Check sheet for the drawn part. Datum: minimum x, y, z corner. Units: mm. A direction names the side the tool comes from. Round coordinates to 2 decimals unless told otherwise and drop trailing zeros. Loops run counter-clockwise (first coordinate to the right, second up) from the corner with the lowest first, then second, coordinate; pieces in that order, holes last. Notation, with made-up numbers: (84.25, 70) - (90.25, 70) arc R27 cw to (90.25, 99) - close; hole circle Ø2 at (86, -19.75). An arc over 180 degrees is marked (long way). Use CSV: the item, a comma, the result in double quotes.
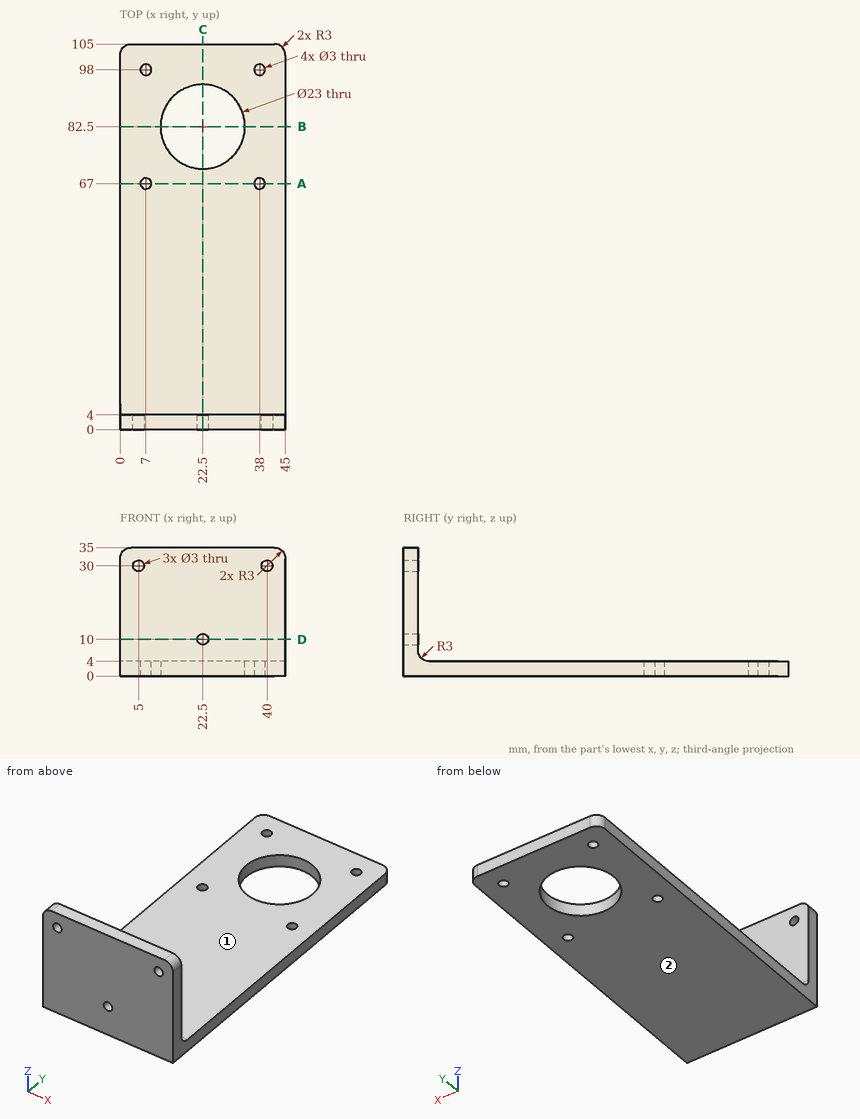
1) Cross-section at D-D, the plane z = 10. Record the cut outline in (x, y), then the cut area to 3 significant figures.
Returned:
outline,"(0, 0) - (21, 0) - (21, 4) - (0, 4) - close; (24, 0) - (45, 0) - (45, 4) - (24, 4) - close"
area,"168 mm²"
2) Access from +Z, -Z, +X, -X, +Y, -Y to the whole of each face (thin tool, end or side, straight path). Record for the marked faces 1 and 2.
Returned:
face 1,"+Z, +X, -X, +Y"
face 2,"-Z, +X, -X, +Y, -Y"
3) Cross-section at C-C, the plane x = 22.5. Record the cut outline in (y, z), then the cut area to 3 significant figures.
Returned:
outline,"(0, 0) - (71, 0) - (71, 4) - (7, 4) arc R3 cw to (4, 7) - (4, 8.5) - (0, 8.5) - close; (0, 11.5) - (4, 11.5) - (4, 35) - (0, 35) - close; (94, 0) - (105, 0) - (105, 4) - (94, 4) - close"
area,"442 mm²"
4) Thickness scan on probe 1 along Y at (x, z) = (38, 2); probe 2 along X at (y, z) = (67, 2.5); probe 3 along Z at (x, y) = (40, 1.05). Record the ranges inside material, lowest first. Write a range as [from, to].
Returned:
probe 1,"y = [0, 65.5], [68.5, 96.5], [99.5, 105]"
probe 2,"x = [0, 5.5], [8.5, 36.5], [39.5, 45]"
probe 3,"z = [0, 28.5], [31.5, 35]"
5) Cross-section at A-A, the plane y = 67. Record the cut outline in (x, z).
Returned:
outline,"(0, 0) - (5.5, 0) - (5.5, 4) - (0, 4) - close; (8.5, 0) - (36.5, 0) - (36.5, 4) - (8.5, 4) - close; (39.5, 0) - (45, 0) - (45, 4) - (39.5, 4) - close"
6) Gauge pin test, flat ends, axial feed: pin 1 Ø4 at (x, y) = (7, 67) entering from +Z; pin 2 Ø12 at (x, y) = (19, 78.5) entering from -Z; pin 3 Ø5 at (x, z) = (40, 30) entering from +Y. Record the tip position at first contact, or that the pin passes through.
Returned:
pin 1,"stops at z = 4"
pin 2,"passes through"
pin 3,"stops at y = 4"
7) Cross-section at B-B, the plane y = 82.5. Record the cut outline in (x, z), then the cut area to 3 significant figures.
Returned:
outline,"(0, 0) - (11, 0) - (11, 4) - (0, 4) - close; (34, 0) - (45, 0) - (45, 4) - (34, 4) - close"
area,"88.0 mm²"
